Check sheet for the drawn part. Datum: minimum x, y, z corner. Units: mm. A direction names the side the tool comes from. Round coordinates to 2 decimals unless told otherwise and drop trailing zeros. Order: outer loops, then holes, each group sorted by start corner. A loop starts at its lowest first (then second) coordinate and runs counter-clockwise, first axis right, second up. Notation, with made-up numbers: (8, 73.5) -> (21, 73.5) arc R13 cw to (21, 85.5) -> close; hole circle Ø8 at (-33, -8). An arc over 180 degrees is marked (long way). Answer in a Markdown table with one row per item.
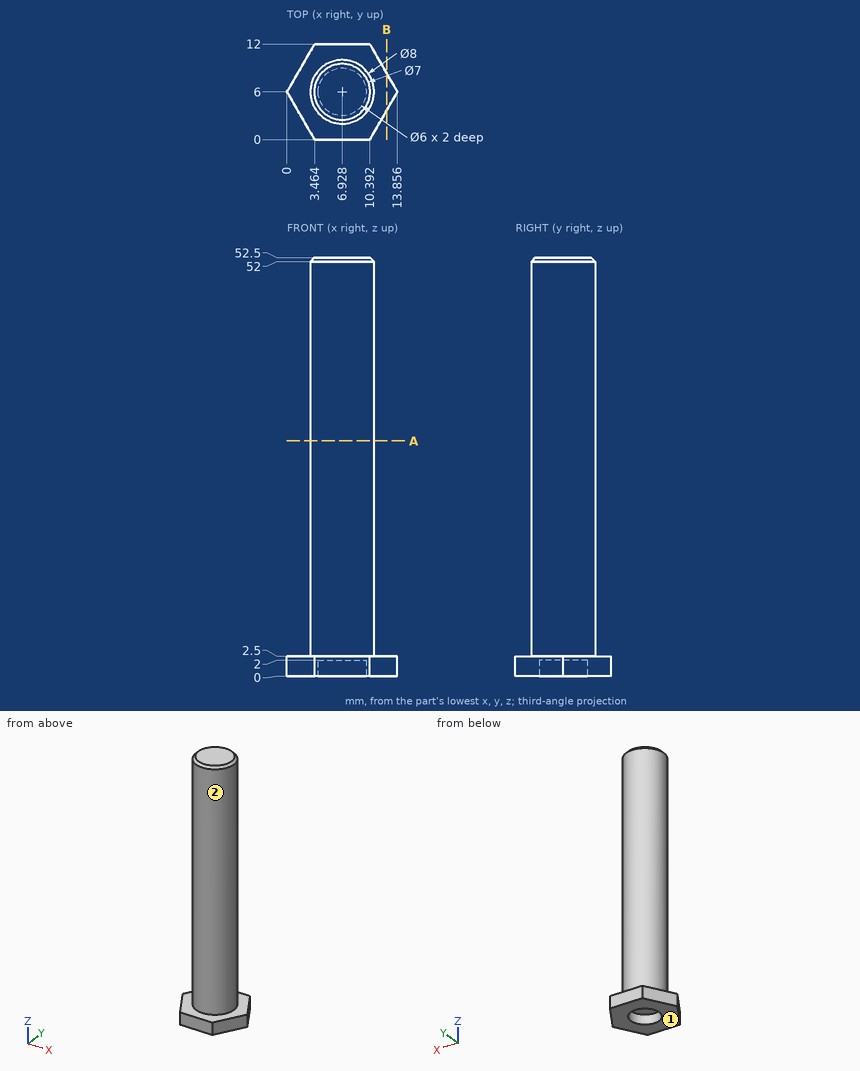
(1) Tool access check on the marked faces 1 and 2. Record the directions out of +Z, -Z, +X, -X, +Y, -Y that give a thin tool (end or side, any length) a straight path to the whole face; none if there is none.
Solutions:
| item | result |
|---|---|
| face 1 | -Z, +X, -X, +Y, -Y |
| face 2 | +Z |
(2) Section check B-B on x = 12.5. Record the boundary of the cut face in (y, z).
Solutions:
| item | result |
|---|---|
| outline | (3.65, 0) -> (8.35, 0) -> (8.35, 2.5) -> (3.65, 2.5) -> close |
(3) Depth check by flat-ended pin: pin 1 Ø6 at (x, y) = (10, 9) entering from +Z; pin 2 Ø3 at (x, z) = (9, 8.5) entering from -Y. Enter the tip coordinate at first touch or a pass-through.
Solutions:
| item | result |
|---|---|
| pin 1 | z = 52.5 |
| pin 2 | y = 2.04 |
(4) Scan lines: probe 1 along Z at (x, y) = (5.5, 8.25); probe 2 along Z at (x, y) = (11.5, 5.5); probe 3 along Y at (x, z) = (8.75, 28). Record each from-to range of solid material in increasing order. Write a range as from..to.
Solutions:
| item | result |
|---|---|
| probe 1 | 2..52.5 |
| probe 2 | 0..2.5 |
| probe 3 | 2.44..9.56 |
(5) Section check A-A on z = 29.5. Record the boundary of the cut face in (x, y).
Solutions:
| item | result |
|---|---|
| outline | circle Ø8 at (6.93, 6) |
